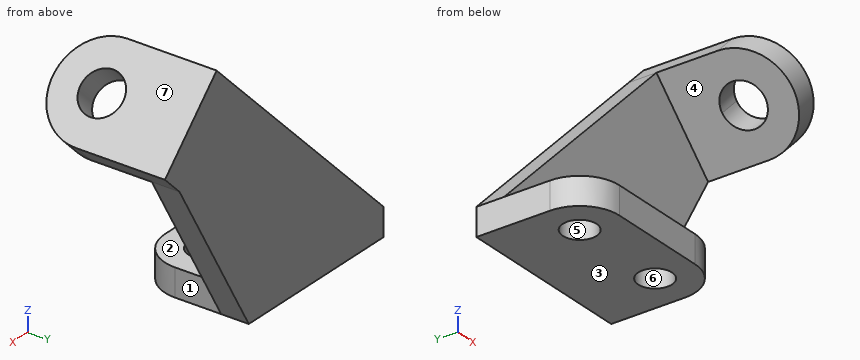
```python
from build123d import *

# Parameters (mm, degrees)
F0_R     = 5.5
F1_DEPTH = 9
F4_DEPTH = 9
F5_DEPTH = 29
F7_DEPTH = 9
F8_DEPTH = 9


with BuildPart() as f1:
    # F0 (on Top) → F1 (new body)
    with BuildSketch(Plane.XY):
        with BuildLine():
            Line((-13, 24), (-13, 0))
            ThreePointArc((-13, 0), (-9.1923881554, -9.1923881554), (0, -13))
            Line((0, -13), (33, -13))
            ThreePointArc((33, -13), (42.1923881554, -9.1923881554), (46, 0))
            Line((46, 0), (46, 24))
            Line((46, 24), (-13, 24))
        make_face()
        Circle(F0_R, mode=Mode.SUBTRACT)
        with BuildLine():
            ThreePointArc((38.5, 0), (33, -5.5), (27.5, 0))
            ThreePointArc((27.5, 0), (33, 5.5), (38.5, 0))
        make_face(mode=Mode.SUBTRACT)
    extrude(amount=F1_DEPTH)

    # F3 (on face) → F4 (join)
    with BuildSketch(Plane(origin=(0, 24, 0), x_dir=(-1, 0, 0), z_dir=(0, 1, 0))):
        Polygon((-65, 64), (-76.313708499, 52.686291501), (-46, 0), (-46, 9), (13, 9), (-53.686291501, 75.313708499), align=None)
    extrude(amount=-F4_DEPTH)

    # F2 (on face) → F5 (join)
    with BuildSketch(Plane(origin=(0, 24, 0), x_dir=(-1, 0, 0), z_dir=(0, 1, 0))):
        Polygon((-76.313708499, 52.686291501), (-65, 64), (-53.686291501, 75.313708499), (-60.0502525317, 81.6776695297), (-82.6776695297, 59.0502525317), align=None)
    extrude(amount=-F5_DEPTH)

    # F6 (on face) → F7 (cut)
    with BuildSketch(Plane(origin=(70.8639610307, 0, 70.8639610307), x_dir=(0, 1, 0), z_dir=(0.7071067812, 0, 0.7071067812))):
        with BuildLine():
            ThreePointArc((2, -0.7071067812), (-0.0502525317, 4.2426406871), (-5, 6.2928932188))
            Line((-5, 6.2928932188), (-5, -7.7071067812))
            ThreePointArc((-5, -7.7071067812), (-0.0502525317, -5.6568542495), (2, -0.7071067812))
        make_face()
    extrude(amount=-F7_DEPTH, mode=Mode.SUBTRACT)

    # F6 (on face) → F8 (join)
    with BuildSketch(Plane(origin=(70.8639610307, 0, 70.8639610307), x_dir=(0, 1, 0), z_dir=(0.7071067812, 0, 0.7071067812))):
        with BuildLine():
            Line((-5, 6.2928932188), (-5, 15.2928932188))
            ThreePointArc((-5, 15.2928932188), (-21, -0.7071067812), (-5, -16.7071067812))
            Line((-5, -16.7071067812), (-5, -7.7071067812))
            ThreePointArc((-5, -7.7071067812), (-12, -0.7071067812), (-5, 6.2928932188))
        make_face()
    extrude(amount=-F8_DEPTH)


solid = f1.part
```
Input: part model. Units: mm. Frame: model coordinates. Face numbers are marked on the shaded views. A direction names the side the tool comes from. Give positions to 0.01 mm unless a question says otherwise; leave off trailing zeros. Order: outer loops, then holes, each group sorted by start corner. A loop starts at its lowest first (then second) coordinate and runs counter-clockwise, first axis right, second up.
1. Mould query, pull axis X, two halves, no side actions, for the marked faces 4, 5, 6 and 7. Classes: released by +X, released by -X, zero draft, split by the parting line, or undercut.
Derived:
face 4: released by -X
face 5: undercut
face 6: undercut
face 7: released by +X
2. Section D-D on x = 15. Return the cut outline in (y, z).
Derived:
outline: (-13, 0) - (24, 0) - (24, 36.84) - (15, 36.84) - (15, 9) - (-13, 9) - close
3. Section B-B on y = -7. Return the cut outline in (x, z), and give its area (3 significant figures).
Derived:
outline: (-10.95, 0) - (43.95, 0) - (43.95, 9) - (-10.95, 9) - close; (53.78, 75.22) - (60.26, 68.74) - (66.62, 75.11) - (60.14, 81.59) - close; (69.74, 59.26) - (76.22, 52.78) - (82.59, 59.14) - (76.11, 65.62) - close
area: 659 mm2
4. Reachability of the marked faces 1, 2 and 3 from +Z, -Z, +X, -X, +Y, -Y: full face, straight path, thin tool, end or side. Return the list, or none.
Derived:
face 1: +Z, -Z, +X, -Y
face 2: +Z, +X, -X, -Y
face 3: -Z, +X, -X, +Y, -Y
5. Pin query (flat end, axial travel): pin 1 (9 mm diameter, centred on x = 33, y = 0, fed in from +Z); pin 2 (6 mm diameter, centred on x = 40, z = 58, fed in from -Y); pin 3 (1 mm diameter, centred on x = 1, y = 9.5, fed in from +Z); pin 4 (7 mm diameter, centred on y = 6, z = 2.5, fed in from +X). Return the tip coordinate at first contact, or that it passes through.
Derived:
pin 1: passes through
pin 2: stops at y = 15
pin 3: stops at z = 9
pin 4: stops at x = 46
6. Section A-A on y = 9. Return the cut outline in (x, z), and give its area (3 significant figures).
Derived:
outline: (-13, 0) - (46, 0) - (46, 9) - (-13, 9) - close; (53.69, 75.31) - (76.31, 52.69) - (82.68, 59.05) - (60.05, 81.68) - close
area: 819 mm2
7. Material intervals for L1, parallel to Y at x = 33, z = 4.75; L2, parallel to Z at x = 31, y = 10.5; L3, parallel to Y at x = 44, z = 41.5, sorted ascending.
Derived:
L1: y = -13 to -5.5, 5.5 to 24
L2: z = 0 to 9
L3: y = 15 to 24
8. Section C-C on x = -3.5. Return the cut outline in (y, z).
Derived:
outline: (-12.52, 0) - (-4.24, 0) - (-4.24, 9) - (-12.52, 9) - close; (4.24, 0) - (24, 0) - (24, 18.45) - (15, 18.45) - (15, 9) - (4.24, 9) - close
